Geometry: final body of the model. Coordinates: model frame, mm. A direction names the side the tool comes from. Give positions to 0.01 mm unless a question says otherwise; leave off trailing zeros. Loops run counter-clockwise (first coordinate to the right, second up) from the corner with the lowest first, then second, coordinate; pieces in that order, holes last. Notation, with made-up numbers: (47.25, 13.25) -> (66.25, 13.25) arc R21 ccw to (66.25, 33.25) -> close; hole circle Ø4 at (67, 84). An arc over 180 degrees is marked (long way). Answer in a Markdown table with one row per item. Add a question column.
from build123d import *

# Parameters (mm, degrees)
SKETCH2_W                    = 39
SKETCH2_H                    = 10
BASE_FLANGE1_DEPTH           = 0.7
EDGE_FLANGE1_STRIP_W         = 4.8
EDGE_FLANGE1_STRIP_H         = 0.7
EDGE_FLANGE1_STRIP_CUT_DEPTH = 10
EDGE_FLANGE1_DEPTH           = 10
EDGE_FLANGE2_STRIP_W         = 4.8
EDGE_FLANGE2_STRIP_H         = 0.7
EDGE_FLANGE2_STRIP_CUT_DEPTH = 10
EDGE_FLANGE2_DEPTH           = 10
FILLET1_R                    = 1


# Sheet-metal steps are written as plain solids
with BuildPart() as part:
    # Sketch2 → Base-Flange1 (new body)
    with BuildSketch(Plane.XY):
        Rectangle(SKETCH2_W, SKETCH2_H)
    extrude(amount=-BASE_FLANGE1_DEPTH)

    # Edge-Flange1 strip (across the edge) → Edge-Flange1 strip cut (cut)
    with BuildSketch(Plane(origin=(-19.5, 5, 0), x_dir=(1, 0, 0), z_dir=(0, -1, 0))):
        with Locations((-1.4, -0.35)):
            Rectangle(EDGE_FLANGE1_STRIP_W, EDGE_FLANGE1_STRIP_H)
    extrude(amount=EDGE_FLANGE1_STRIP_CUT_DEPTH, mode=Mode.SUBTRACT)

    # Edge-Flange1 section (across the edge) → Edge-Flange1 (add)
    with BuildSketch(Plane(origin=(-19.5, 5, 0), x_dir=(1, 0, 0), z_dir=(0, -1, 0))):
        with BuildLine():
            Line((-0.7, 1), (-0.7, 8.3))
            Line((-0.7, 8.3), (0, 8.3))
            Line((0, 8.3), (0, 1))
            ThreePointArc((0, 1), (0.292893219, 0.292893219), (1, 0))
            Line((1, 0), (1, -0.7))
            ThreePointArc((1, -0.7), (-0.202081528, -0.202081528), (-0.7, 1))
        make_face()
    extrude(amount=EDGE_FLANGE1_DEPTH)

    # Edge-Flange2 strip (across the edge) → Edge-Flange2 strip cut (cut)
    with BuildSketch(Plane(origin=(19.5, -5, 0), x_dir=(-1, 0, 0), z_dir=(0, 1, 0))):
        with Locations((-1.4, -0.35)):
            Rectangle(EDGE_FLANGE2_STRIP_W, EDGE_FLANGE2_STRIP_H)
    extrude(amount=EDGE_FLANGE2_STRIP_CUT_DEPTH, mode=Mode.SUBTRACT)

    # Edge-Flange2 section (across the edge) → Edge-Flange2 (add)
    with BuildSketch(Plane(origin=(19.5, -5, 0), x_dir=(-1, 0, 0), z_dir=(0, 1, 0))):
        with BuildLine():
            Line((-0.7, 1), (-0.7, 8.3))
            Line((-0.7, 8.3), (0, 8.3))
            Line((0, 8.3), (0, 1))
            ThreePointArc((0, 1), (0.292893219, 0.292893219), (1, 0))
            Line((1, 0), (1, -0.7))
            ThreePointArc((1, -0.7), (-0.202081528, -0.202081528), (-0.7, 1))
        make_face()
    extrude(amount=EDGE_FLANGE2_DEPTH)

    # Fillet1
    fillet1_edges = [part.edges().sort_by_distance(p)[0] for p in [
        (-19.85, 5, 8.3),
        (-19.85, -5, 8.3),
        (19.85, -5, 8.3),
        (19.85, 5, 8.3),
    ]]
    fillet(fillet1_edges, radius=FILLET1_R)


solid = part.part
(1) Cut plane C-C on x = 16.5. Return the cut outline in (y, z), then the cut area to 3 significant figures.
(2) Material intervals for line 1 along X through (y, z) = (2.25, 3); line 2 along Z through (x, y) = (-18, 2); line 3 along X through (y, z) = (3, 0.5), sorted ascending. Write a range as from..to.
(3) Cut plane B-B on y = -2. Return the cut outline in (x, z).
(4) Cut plane A-A on z = 3.75. Return the cut outline in (x, y), then the cut area to 3 significant figures.
(5) Draft query along X for faces 3 (the cylindrical face through (19.689, -0.07, -0.215)), 4 (the flat face through (-6.1, 5, -0.2)), 5 (the flat face through (-19.5, 0, 5)), 6 (the cylindrical face through (-19.689, 0.07, -0.215)). Return one class per face: +X half, -X half, draft (parallel to the pull), parting line (faces both ways), or undercut.
(6) Reachability of faces 1 (the cylindrical face through (-19.215, 0.07, 0.301)), 2 (the flat face through (0, 0, -0.7)) from +Z, -Z, +X, -X, +Y, -Y: full face, straight path, thin tool, end or side. Return the list, or none.
(7) Pin query (flat end, axial travel): pin 1 Ø4 at (x, y) = (6, 3.5) entering from +Z. Return the tip coordinate at first contact, or that it passes through.
Answer list:
| question | item | result |
|---|---|---|
| 1 | outline | (-5, -0.7) -> (5, -0.7) -> (5, 0) -> (-5, 0) -> close |
| 1 | area | 7.00 mm² |
| 2 | line 1 | x = -20.2..-19.5, 19.5..20.2 |
| 2 | line 2 | z = -0.7..0 |
| 2 | line 3 | x = -20.12..-19.37, 19.37..20.12 |
| 3 | outline | (-20.2, 1) arc R1.7 ccw to (-18.5, -0.7) -> (18.5, -0.7) arc R1.7 ccw to (20.2, 1) -> (20.2, 8.3) -> (19.5, 8.3) -> (19.5, 1) arc R1 cw to (18.5, 0) -> (-18.5, 0) arc R1 cw to (-19.5, 1) -> (-19.5, 8.3) -> (-20.2, 8.3) -> close |
| 4 | outline | (-20.2, -5) -> (-19.5, -5) -> (-19.5, 5) -> (-20.2, 5) -> close; (19.5, -5) -> (20.2, -5) -> (20.2, 5) -> (19.5, 5) -> close |
| 4 | area | 14.0 mm² |
| 5 | face 3 | +X half |
| 5 | face 4 | draft |
| 5 | face 5 | undercut |
| 5 | face 6 | -X half |
| 6 | face 1 | +Z, +Y, -Y |
| 6 | face 2 | -Z, +X, -X, +Y, -Y |
| 7 | pin 1 | stops at z = 0 |
